from build123d import *

# Parameters (mm, degrees)
SKETCH1_W           = 23
SKETCH1_H           = 3.6
BOSS_EXTRUDE1_DEPTH = 1
SKETCH2_W           = 1
SKETCH2_H           = 3.6
BOSS_EXTRUDE2_DEPTH = 2.4
SKETCH3_W           = 1
SKETCH3_H           = 1.2
BOSS_EXTRUDE3_DEPTH = 3.6
FILLET1_SIZE        = 0.6
FILLET2_R           = 0.6
FILLET3_R           = 0.4


with BuildPart() as part:
    # Sketch1 → Boss-Extrude1 (new body)
    with BuildSketch(Plane(origin=(0, 0, 0), x_dir=(1, 0, 0), z_dir=(0, 1, 0))):
        with Locations((11.5, -1.8)):
            Rectangle(SKETCH1_W, SKETCH1_H)
    extrude(amount=BOSS_EXTRUDE1_DEPTH)

    # Sketch2 → Boss-Extrude2 (add)
    with BuildSketch(Plane(origin=(0, 1, 0), x_dir=(1, 0, 0), z_dir=(0, 1, 0))):
        with Locations((0.5, -1.8)):
            Rectangle(SKETCH2_W, SKETCH2_H)
        with Locations((22.5, -1.8)):
            Rectangle(SKETCH2_W, SKETCH2_H)
    extrude(amount=BOSS_EXTRUDE2_DEPTH)

    # Sketch3 → Boss-Extrude3 (add)
    with BuildSketch(Plane.XY.offset(3.6)):
        with Locations((1.5, 2.8)):
            Rectangle(SKETCH3_W, SKETCH3_H)
        with Locations((21.5, 2.8)):
            Rectangle(SKETCH3_W, SKETCH3_H)
    extrude(amount=-BOSS_EXTRUDE3_DEPTH)

    # Fillet1
    # a fillet whose section is not a circle: 0.6 mm, written as the material it takes off along each edge
    with BuildSketch(Plane(origin=(21, 3.4, 5.1), x_dir=(1, 0, 0), z_dir=(0, 0, -1)), Plane(origin=(2, 3.4, 5.1), x_dir=(0, -1, 0), z_dir=(0, 0, -1))) as fillet1_piece_1:
        with BuildLine():
            Bezier((FILLET1_SIZE, 0), (0, 0), (0, FILLET1_SIZE), weights=[1, 0.052631579, 1])
            Line((0, FILLET1_SIZE), (0, 0))
            Line((0, 0), (FILLET1_SIZE, 0))
        make_face()
    extrude(amount=6.6, mode=Mode.SUBTRACT)

    # Fillet2
    fillet2_edges = [part.edges().sort_by_distance(p)[0] for p in [
        (23, 0, 1.8),
        (0, 0, 1.8),
    ]]
    fillet(fillet2_edges, radius=FILLET2_R)

    # Fillet3
    fillet3_edges = [part.edges().sort_by_distance(p)[0] for p in [
        (11.5, 1, 3.6),
        (11.5, 1, 0),
    ]]
    fillet(fillet3_edges, radius=FILLET3_R)


solid = part.part
The model under review builds one solid part; all positions refer to its coordinate system, in mm. A direction names the side the tool comes from. Round coordinates to 2 decimals unless told otherwise and drop trailing zeros. Loops run counter-clockwise (first coordinate to the right, second up) from the corner with the lowest first, then second, coordinate; pieces in that order, holes last. Notation, with made-up numbers: M 50.5,7.5 L 89.5,7.5 A7 cw 89.5,13.5 Z; hole C 85,73 d8. An arc over 180 degrees is marked long. Answer as CSV lines item,"result".
1. Draft analysis for pull direction X (two halves, no side actions). For faces 1 (the face through (11.4, 0.4, 0)), 2 (the face through (0, 2, 2)), 3 (the face through (21.5, 2.2, 1.8)), state which applies: pulls with the +X half, pulls with the -X half, needs draft (parallel to the pull), parting line crosses it, or undercut.
Outcome:
face 1,"needs draft"
face 2,"pulls with the -X half"
face 3,"undercut"
2. Insertion check: pin 1 Ø1.4 at (x, z) = (15, 2) entering from +Y. The pin has a flat end and moves straight along its axis. Give the tip position at first contact, or say it passes through.
Outcome:
pin 1,"stops at y = 1"
3. We need section A-A (y = 1.6). Give the boundary of the cut face in (x, z), plus the area to 3 significant figures.
Outcome:
outline,"M 0,0 L 1,0 L 1,3.6 L 0,3.6 Z; M 22,0 L 23,0 L 23,3.6 L 22,3.6 Z"
area,"7.20 mm2"
4. For faces 4 (the face through (1.5, 2.2, 1.8)), 5 (the face through (11.4, 0.4, 3.6)), list the 3-axis set-ups (+Z, -Z, +X, -X, +Y, -Y) from which the entire face can be reached by the end or side of a thin tool; tool diameter is ignored.
Outcome:
face 4,"+Z, -Z"
face 5,"+Z, +X, -X, +Y, -Y"
5. To check wall thickness, follow L1, parallel to X at y = 1.65, z = 3.45; L2, parallel to Y at x = 6.25, z = 0.7; L3, parallel to X at y = 3.1, z = 0.75. State the ranges of each line that lie inside material, in increasing order. Write a range as [from, to].
Outcome:
L1,"x = [0, 1], [22, 23]"
L2,"y = [0, 1]"
L3,"x = [0, 1.73], [21.27, 23]"
6. We need section B-B (x = 3.75). Give the boundary of the cut face in (y, z).
Outcome:
outline,"M 0,0 L 0.6,0 A0.4 ccw 1,0.4 L 1,3.2 A0.4 ccw 0.6,3.6 L 0,3.6 Z"
